Verification items for this drawing (mm, ordinates from the low corner). Round coordinates to 2 decimals unless told otherwise and drop trailing zeros. Loops run counter-clockwise (first coordinate to the right, second up) from the corner with the lowest first, then second, coordinate; pieces in that order, holes last. Notation, with made-up numbers: (33, 65) - (46, 65) arc R24 cw to (46, 75) - close; hole circle Ø9 at (24, -24.75). An arc over 180 degrees is marked (long way). Answer in a Markdown table with one row per item. Add a question column.
(1) Cross-section at C-C on x = 19.5. Enter the section's corners in (y, z).
(2) Thickness scan on line 1 along X through (y, z) = (41, 2.15); line 2 along X through (y, z) = (31, 3.9); line 3 along Y through (x, z) = (41.5, 0.4) (1 decimal). Record the ranges inside material, lowest first.
(3) Cross-section at A-A on z = 3.8. Enter the section's corners in (x, y).
(4) Cross-section at D-D on y = 13. Enter the section's corners in (x, z), then the cut area to 3 significant figures.
(5) Gauge pin test, flat ends, axial feed: pin 1 (2.5 mm diameter, centred on y = 34.5, z = 3.5, fed in from +X); pin 2 (1.5 mm diameter, centred on x = 67.5, z = 3.5, fed in from +Y) (1 decimal); pin 3 (1.5 mm diameter, centred on x = 67.5, z = 3, fed in from -Y). Record the tip position at first contact, or that the pin passes through.
(6) Cross-section at B-B on y = 34. Enter the section's corners in (x, z).
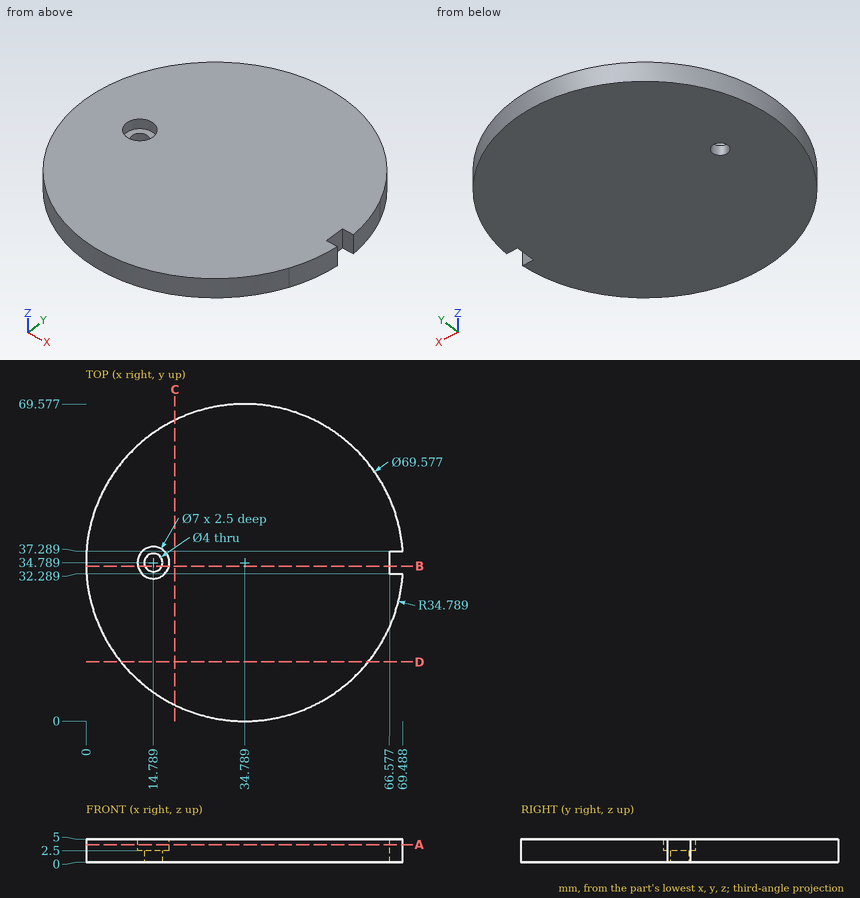
Answers:
| question | item | result |
|---|---|---|
| 1 | outline | (3.54, 0) - (66.04, 0) - (66.04, 5) - (3.54, 5) - close |
| 2 | line 1 | x = 0.56 to 69.02 |
| 2 | line 2 | x = 0.21 to 69.37 |
| 2 | line 3 | y = 0.7 to 68.9 |
| 3 | outline | (66.58, 20.66) arc R34.79 ccw to (69.49, 32.29) - (66.58, 32.29) - (66.58, 37.29) - (69.49, 37.29) arc R34.79 ccw to (66.58, 48.92) arc R34.79 ccw (long way) to start; hole circle Ø7 at (14.79, 34.79) |
| 4 | outline | (7.67, 0) - (61.91, 0) - (61.91, 5) - (7.67, 5) - close |
| 4 | area | 271 mm^2 |
| 5 | pin 1 | stops at x = 66.58 |
| 5 | pin 2 | stops at y = 48.5 |
| 5 | pin 3 | stops at y = 21.05 |
| 6 | outline | (0.01, 0) - (12.95, 0) - (12.95, 2.5) - (11.38, 2.5) - (11.38, 5) - (0.01, 5) - close; (16.63, 0) - (66.58, 0) - (66.58, 5) - (18.2, 5) - (18.2, 2.5) - (16.63, 2.5) - close |
